```python
from build123d import *

# Parameters (mm, degrees)
SKETCH1_W           = 88.9
SKETCH1_H           = 90
BASE_DEPTH          = 2
SKETCH2_W           = 63.5
SKETCH2_H           = 6
FACE_PLATE_DEPTH    = 117
SKETCH5_R           = 10.5
SKETCH5_R_2         = 1.6
FACE_HOLES_DEPTH    = 138.261802771
FILLET2_R           = 10
FILLET3_R           = 20
SKETCH23_W          = 55
SKETCH23_H          = 117
CUT_EXTRUDE6_DEPTH  = 4
FILLET4_R           = 110
SKETCH24_W          = 88.9
SKETCH24_H          = 46
CUT_EXTRUDE7_DEPTH  = 3
SKETCH25_R          = 1.55
CUT_EXTRUDE8_DEPTH  = 134.003016883
CUT_EXTRUDE9_DEPTH  = 134.003016883
FILLET5_R           = 3
CUT_EXTRUDE10_DEPTH = 134.793880741


with BuildPart() as part:
    # Sketch1 → Base (new body)
    with BuildSketch(Plane(origin=(0, 0, 0), x_dir=(1, 0, 0), z_dir=(0, 1, 0))):
        Rectangle(SKETCH1_W, SKETCH1_H)
    extrude(amount=BASE_DEPTH)

    # Sketch2 → Face Plate (add)
    with BuildSketch(Plane(origin=(0, 2, 0), x_dir=(1, 0, 0), z_dir=(0, 1, 0))):
        with Locations((0, -4)):
            Rectangle(SKETCH2_W, SKETCH2_H)
    extrude(amount=FACE_PLATE_DEPTH)

    # Sketch5 → Face Holes (cut, through all)
    with BuildSketch(Plane.XY.offset(7)):
        with Locations((0, 97)):
            Circle(SKETCH5_R)
        with Locations((12.990381057, 89.5)):
            Circle(SKETCH5_R_2)
        with Locations((-12.990381057, 89.5)):
            Circle(SKETCH5_R_2)
        with Locations((0, 112)):
            Circle(SKETCH5_R_2)
        with BuildLine():
            Line((-9.7, 7), (-9.7, 29))
            ThreePointArc((-9.7, 29), (-8.35, 30.35), (-7, 29))
            Line((-7, 29), (-7, 7))
            ThreePointArc((-7, 7), (-8.35, 5.65), (-9.7, 7))
        make_face()
        with BuildLine():
            Line((9.7, 29), (9.7, 7))
            ThreePointArc((9.7, 7), (8.35, 5.65), (7, 7))
            Line((7, 7), (7, 29))
            ThreePointArc((7, 29), (8.35, 30.35), (9.7, 29))
        make_face()
        with BuildLine():
            Line((-5, 7), (-5, 29))
            ThreePointArc((-5, 29), (0, 34), (5, 29))
            Line((5, 29), (5, 7))
            ThreePointArc((5, 7), (0, 2), (-5, 7))
        make_face()
    extrude(amount=-FACE_HOLES_DEPTH, mode=Mode.SUBTRACT)

    # Fillet2
    fillet2_edges = [part.edges().sort_by_distance(p)[0] for p in [
        (-44.45, 1, -45),
        (44.45, 1, -45),
        (44.45, 1, 45),
        (-44.45, 1, 45),
    ]]
    fillet(fillet2_edges, radius=FILLET2_R)

    # Fillet3
    fillet3_edges = [part.edges().sort_by_distance(p)[0] for p in [
        (-31.75, 119, 4),
        (31.75, 119, 4),
    ]]
    fillet(fillet3_edges, radius=FILLET3_R)

    # Sketch23 → Cut-Extrude6 (cut)
    with BuildSketch(Plane.XY.offset(7)):
        with Locations((0, 60.5)):
            Rectangle(SKETCH23_W, SKETCH23_H)
    extrude(amount=-CUT_EXTRUDE6_DEPTH, mode=Mode.SUBTRACT)

    # Fillet4
    # the kernel refuses this fillet: 110 mm, written as the material it adds along each edge
    with BuildSketch(Plane(origin=(-180.406228863, 2, 7), x_dir=(0, 0, 1), z_dir=(1, 0, 0))) as fillet4_piece_1_section:
        with BuildLine():
            CenterArc((110, -83.162491545), FILLET4_R, 130.885192893, 49.114807107)
            Line((0, -83.162491545), (0, 0))
            Line((0, 0), (38, 0))
        make_face()
    fillet4_piece_1 = extrude(amount=420.062457726, mode=Mode.PRIVATE)
    fillet4_piece_1 = split(fillet4_piece_1, bisect_by=Plane(origin=(-31.75, 51.263709825, 12.122352248), z_dir=(1, 0, 0)), keep=Keep.TOP, mode=Mode.PRIVATE)
    fillet4_piece_1 = split(fillet4_piece_1, bisect_by=Plane(origin=(-27.5, 51.263709825, 12.122352248), z_dir=(-1, 0, 0)), keep=Keep.TOP, mode=Mode.PRIVATE)
    add(fillet4_piece_1)
    with BuildSketch(Plane(origin=(27.5, 2, 7), x_dir=(0, 0, 1), z_dir=(1, 0, 0)), Plane(origin=(-31.75, 2, 7), x_dir=(0, 0, 1), z_dir=(1, 0, 0))) as fillet4_piece_2:
        with BuildLine():
            CenterArc((110, -83.162491545), FILLET4_R, 130.885192893, 49.114807107)
            Line((0, -83.162491545), (0, 0))
            Line((0, 0), (38, 0))
        make_face()
    extrude(amount=4.25)
    with BuildSketch(Plane(origin=(-239.656228863, 2, 7), x_dir=(0, 0, 1), z_dir=(1, 0, 0))) as fillet4_piece_3_section:
        with BuildLine():
            CenterArc((110, -83.162491545), FILLET4_R, 130.885192893, 49.114807107)
            Line((0, -83.162491545), (0, 0))
            Line((0, 0), (38, 0))
        make_face()
    fillet4_piece_3 = extrude(amount=420.062457726, mode=Mode.PRIVATE)
    fillet4_piece_3 = split(fillet4_piece_3, bisect_by=Plane(origin=(31.75, 51.263709825, 12.122352248), z_dir=(-1, 0, 0)), keep=Keep.TOP, mode=Mode.PRIVATE)
    fillet4_piece_3 = split(fillet4_piece_3, bisect_by=Plane(origin=(27.5, 51.263709825, 12.122352248), z_dir=(1, 0, 0)), keep=Keep.TOP, mode=Mode.PRIVATE)
    add(fillet4_piece_3)

    # Sketch24 → Cut-Extrude7 (cut)
    with BuildSketch(Plane(origin=(0, 2, 0), x_dir=(1, 0, 0), z_dir=(0, 1, 0))):
        with Locations((0, 22)):
            Rectangle(SKETCH24_W, SKETCH24_H)
    extrude(amount=-CUT_EXTRUDE7_DEPTH, mode=Mode.SUBTRACT)

    # Sketch25 → Cut-Extrude8 (cut, through all)
    with BuildSketch(Plane(origin=(0, 2, 0), x_dir=(1, 0, 0), z_dir=(0, 1, 0))):
        with Locations(Location((38.45, -25, 0), (0, 0, 270))):
            Circle(SKETCH25_R)
        with Locations(Location((-38.45, -25, 0), (0, 0, 270))):
            Circle(SKETCH25_R)
    extrude(amount=-CUT_EXTRUDE8_DEPTH, mode=Mode.SUBTRACT)

    # Sketch26 → Cut-Extrude9 (cut, through all)
    with BuildSketch(Plane(origin=(0, 2, 0), x_dir=(1, 0, 0), z_dir=(0, 1, 0))):
        with BuildLine():
            Line((-27.5, -45), (27.5, -45))
            ThreePointArc((27.5, -45), (0, -22.267826876), (-27.5, -45))
        make_face()
    extrude(amount=-CUT_EXTRUDE9_DEPTH, mode=Mode.SUBTRACT)

    # Fillet5
    fillet5_edges = [part.edges().sort_by_distance(p)[0] for p in [
        (27.5, 56.663146518, 3),
        (-27.5, 56.663146518, 3),
    ]]
    fillet(fillet5_edges, radius=FILLET5_R)

    # Sketch27 → Cut-Extrude10 (cut, through all)
    with BuildSketch(Plane.XY.offset(3)):
        Polygon((0, 45.56624327), (12.5, 52.783121635), (12.5, 67.216878365), (0, 74.43375673), (-12.5, 67.216878365), (-12.5, 52.783121635), align=None)
    extrude(amount=-CUT_EXTRUDE10_DEPTH, mode=Mode.SUBTRACT)


solid = part.part
```
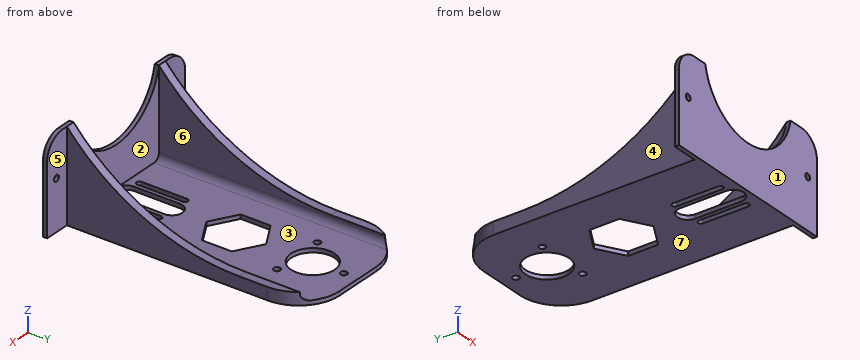
Work out the finished part from the listing and answer in its coordinate system (mm). Face numbers are marked on the shaded views. A direction names the side the tool comes from. Coordinates: 2 decimals unless noted, no trailing zeros. Write each loop counter-clockwise with the first axis right and the second up, starting at its lowest first coordinate (ties: lowest second). Pieces come first, ordered by that corner, then holes.
Q1. A cutting plane is placed at C-C, the plane x = 38.45. Give the vertices of the cut face in (y, z), then the cut area to 3 significant figures.
Q2. Which of the six approach directions +Z, -Z, +X, -X, +Y, -Y give full straight-line access (tool end or side, diameter ignored) to the marked faces 5, 6 and 7?
Q3. Find the intervals of material crossed by line 1 (Y direction, x = 0, z = 1.65); line 2 (X direction, y = 89, z = 2); line 3 (X direction, y = 20.5, z = 20), in increasing order.
Q4. A cutting plane is placed at B-B, the plane y = 70. Give the vertices of the cut face in (x, z), then the cut area to 3 significant figures.
Q5. Each of these flat-tipped pins is pushed along its axis until it touches: pin 1 Ø8 at (x, z) = (24, 7.5) entering from +Y; pin 2 Ø2 at (x, z) = (25, 38.5) entering from -Y; pin 3 Ø1 at (y, z) = (14.5, 2) entering from +X; pin 4 Ø2 at (y, z) = (59, 2) entering from -X. Where does it stop, or does it pass through?
Q6. A cutting plane is placed at A-A, the plane z = 37.5. Give the vertices of the cut face in (x, y), then the cut area to 3 significant figures.
Q7. Determine the mould class of the marked faces 1, 2, 3 and 4 for opening direction X: released by +X, released by -X, zero draft, split by the parting line, or undercut.
Q8. A cutting plane is placed at D-D, the plane y = 89.5. Give the vertices of the cut face in (x, z), then the cut area to 3 significant figures.
Findings below:
1. outline: (0, 1) - (2, 1) - (2, 23.45) - (0, 23.45) - close; (0, 26.55) - (2, 26.55) - (2, 44.17) - (0, 44.17) - close
1. area: 80.1 mm2
2. face 5: +Z, -Z, +X, +Y
2. face 6: +Z, +Y
2. face 7: -Z, +X, -X, +Y, -Y
3. line 1: y = 0 to 2, 34 to 45.57, 74.43 to 86.5, 107.5 to 110.4, 113.6 to 119
3. line 2: x = -31.75 to -14.51, -11.47 to -6.8, 6.8 to 11.47, 14.51 to 31.75
3. line 3: x = -31.75 to -27.5, 27.5 to 31.75
4. outline: (-31.75, 1) - (-7.68, 1) - (-7.68, 3) - (-24.5, 3) arc R3 cw to (-27.5, 6) - (-27.5, 8.05) - (-31.75, 8.05) - close; (7.68, 1) - (31.75, 1) - (31.75, 8.05) - (27.5, 8.05) - (27.5, 6) arc R3 cw to (24.5, 3) - (7.68, 3) - close
4. area: 143 mm2
5. pin 1: stops at y = 111.38
5. pin 2: stops at y = 0
5. pin 3: stops at x = 31.75
5. pin 4: stops at x = -31.75
6. outline: (-44.13, 0) - (-24.92, 0) - (-24.92, 2) - (-27.5, 2) - (-27.5, 9.14) - (-31.75, 9.14) - (-31.75, 2) - (-44.13, 2) - close; (24.92, 0) - (44.13, 0) - (44.13, 2) - (31.75, 2) - (31.75, 9.14) - (27.5, 9.14) - (27.5, 2) - (24.92, 2) - close
6. area: 138 mm2
7. face 1: zero draft
7. face 2: undercut
7. face 3: undercut
7. face 4: released by -X
8. outline: (-31.75, 1) - (-14.59, 1) - (-14.59, 3) - (-24.5, 3) arc R3 cw to (-27.5, 6) - (-27.5, 7) - (-31.75, 7) - close; (-11.39, 1) - (-7.35, 1) - (-7.35, 3) - (-11.39, 3) - close; (7.35, 1) - (11.39, 1) - (11.39, 3) - (7.35, 3) - close; (14.59, 1) - (31.75, 1) - (31.75, 7) - (27.5, 7) - (27.5, 6) arc R3 cw to (24.5, 3) - (14.59, 3) - close
8. area: 123 mm2
